```python
from build123d import *

# Parameters (mm, degrees)
MAKAS_BA_LANT_S_DEPTH    = 60
MOTOR_UZANT_S_DEPTH      = 15
MOTOR_UZANT_S_DEPTH_BACK = 15
IZIM3_R                  = 1.5
C_VATALAR_DEPTH          = 112.018016714


# Read off the part's stored shape, not the designer's step: makas bağlantısı
with BuildPart() as part:
    # makas bağlantısı outline → makas bağlantısı (new body)
    with BuildSketch(Plane(origin=(0, 0, 0), x_dir=(1, 0, 0), z_dir=(0, 1, 0))):
        Polygon((-5, 5), (-5, 20), (-10, 20), (-10, 10), (-15, 10), (-15, -10), (15, -10), (15, 10), (10, 10), (10, 20), (5, 20), (5, 5), (10, 5), (10, -5), (-10, -5), (-10, 5), align=None)
    extrude(amount=MAKAS_BA_LANT_S_DEPTH)

    # Çizim2 → motor uzantısı (add, two sides: drawn at the far end of the back side and taken through both)
    with BuildSketch(Plane(origin=(0, 0, 0), x_dir=(0, 0, -1), z_dir=(1, 0, 0)).offset(-MOTOR_UZANT_S_DEPTH_BACK)):
        with BuildLine():
            Line((-10, 60), (-90, 60))
            Line((-90, 60), (-90, 50))
            add(Edge.make_bspline(
                [(-10, 0), (-10, 50), (-90, 50)],
                knots=[0, 0, 0, 1.570796327, 1.570796327, 1.570796327], degree=2, weights=[1, 0.707106781, 1]))
            Line((-10, 0), (-10, 60))
        make_face()
    extrude(amount=MOTOR_UZANT_S_DEPTH + MOTOR_UZANT_S_DEPTH_BACK)

    # Çizim3 → cıvatalar (cut, through all)
    with BuildSketch(Plane.ZY.offset(10)):
        with Locations((-15, 50.141064744)):
            Circle(IZIM3_R)
        with Locations((-15, 8.810242757)):
            Circle(IZIM3_R)
    extrude(amount=-C_VATALAR_DEPTH, mode=Mode.SUBTRACT)


solid = part.part
```
Read the model definition and answer for the solid it produces. Units are mm, in the model's axes. A direction names the side the tool comes from. Give positions to 0.01 mm unless a question says otherwise; leave off trailing zeros. Write each loop counter-clockwise with the first axis right and the second up, starting at its lowest first coordinate (ties: lowest second). Pieces come first, ordered by that corner, then holes. Notation, with made-up numbers: M 52,-19.5 L 70,-19.5 A8 ccw 70,-12.5 Z; hole C 66,-27.5 d8. An arc over 180 degrees is marked long. Put each result on its own line as item: value. Start each with the question number.
1. Consider line 1 along Y through (x, z) = (6, -15); line 2 along X through (y, z) = (22.5, 2); line 3 along X through (y, z) = (26, -13.5). Determine where each line is inside the solid, lowest interval first.
2. The part is cut by section D-D, the plane x = -8. Give the number of separate pieces and of enclosed holes in the cut face, and give its area (3 significant figures).
3. The part is cut by section A-A, the plane z = -15. Give the vertices of the cut face in (x, y).
4. The part is cut by section B-B, the plane z = 0.5. Give the vertices of the cut face in (x, y), and give its area (3 significant figures).
5. Each of these flat-tipped pins is pushed along its axis until it touches: pin 1 Ø4 at (x, y) = (-11.5, 40.5) entering from -Z; pin 2 Ø2 at (x, z) = (9.5, 57.5) entering from -Y; pin 3 Ø2.5 at (y, z) = (8.81, -15) entering from -X; pin 4 Ø8 at (x, z) = (8.5, 76) entering from -Y. Where does it stop, or does it pass through?
6. Which of the six approach directions +Z, -Z, +X, -X, +Y, -Y give full straight-line access (tool end or side, diameter ignored) to faces 1 (the flat face through (0, 60, 46)), 2 (the flat face through (10, 30, -15)), 3 (the flat face through (-12, 30, -10)), 4 (the flat face through (-5, 30, -12)), 5 (the flat face through (7, 30, -5))?
7. The part is cut by section C-C, the plane y = 56.5. Give the vertices of the cut face in (x, z).
8. For a pull along X with two mould halves and no side action, classify faces 6 (the cylindrical face through (7.46, 8.88, -16.5)), 7 (the flat face through (-15, 37, 18)), 8 (the flat face through (-8, 30, -5)) as released by +X, released by -X, zero draft, split by the parting line, or undercut.
Final values:
1. line 1: y = 0 to 7.31, 10.31 to 48.64, 51.64 to 60
1. line 2: x = -15 to -10, 10 to 15
1. line 3: x = -10 to -5, 5 to 10
2. separate pieces: 2
2. enclosed holes: 2
2. area: 2,840 mm²
3. outline: M -10,0 L -5,0 L -5,7.31 L -10,7.31 Z; M -10,10.31 L -5,10.31 L -5,48.64 L -10,48.64 Z; M -10,51.64 L -5,51.64 L -5,60 L -10,60 Z; M 5,0 L 10,0 L 10,7.31 L 5,7.31 Z; M 5,10.31 L 10,10.31 L 10,48.64 L 5,48.64 Z; M 5,51.64 L 10,51.64 L 10,60 L 5,60 Z
4. outline: M -15,0 L -10,0 L -10,60 L -15,60 Z; M 10,0 L 15,0 L 15,60 L 10,60 Z
4. area: 600 mm²
5. pin 1: stops at z = -20
5. pin 2: stops at y = 45.41
5. pin 3: passes through
5. pin 4: stops at y = 48.72
6. face 1: +Z, -Z, +X, -X, +Y
6. face 2: -Z, +X, +Y, -Y
6. face 3: -Z, -X, +Y, -Y
6. face 4: -Z, +Y, -Y
6. face 5: +Y, -Y
7. outline: M -15,-10 L -10,-10 L -10,-20 L -5,-20 L -5,-5 L -10,-5 L -10,5 L 10,5 L 10,-5 L 5,-5 L 5,-20 L 10,-20 L 10,-10 L 15,-10 L 15,90 L -15,90 Z
8. face 6: zero draft
8. face 7: released by -X
8. face 8: undercut
